Build history of the part. All positions in model axes, mm. Coordinates: 2 decimals unless noted, no trailing zeros. Order: outer loops, then holes, each group sorted by start corner. A loop starts at its lowest first (then second) coordinate and runs counter-clockwise, first axis right, second up. Notation, with made-up numbers: (-18.5, 31.25) - (-13.5, 31.25) arc R16 ccw to (-13.5, 39.25) - close; hole circle Ø11 at (14, 80). An arc over 180 degrees is marked (long way). Write each question's results on one line, items separated by ' | '.
from build123d import *

# Parameters (mm, degrees)
F0_W     = 152.4
F0_H     = 76.2
F1_DEPTH = 1.5875
F2_W     = 5.08
F2_H     = 50.8
F3_DEPTH = 25.4
F5_DEPTH = 25.4


# Not quite as in the source:
# - a length typed as a fraction of an inch, garbled in the dataset ("3 / 203.2 mm" for 3/8 in), is restored


with BuildPart() as f1:
    # F0 (on Front) → F1 (new body)
    with BuildSketch(Plane.XZ):
        Rectangle(F0_W, F0_H)
    extrude(amount=F1_DEPTH)

    # F2 (on face) → F3 (cut)
    with BuildSketch(Plane.XZ.offset(1.5875)):
        Rectangle(F2_W, F2_H)
    extrude(amount=-F3_DEPTH, mode=Mode.SUBTRACT)

    # F4 (on face) → F5 (cut)
    with BuildSketch(Plane.XZ.offset(1.5875)):
        with BuildLine():
            Line((2.54, -25.4), (-2.54, -25.4))
            ThreePointArc((-2.54, -25.4), (0, -27.94), (2.54, -25.4))
        make_face()
        with BuildLine():
            ThreePointArc((2.54, 25.4), (0, 27.94), (-2.54, 25.4))
            Line((-2.54, 25.4), (2.54, 25.4))
        make_face()
    extrude(amount=-F5_DEPTH, mode=Mode.SUBTRACT)


solid = f1.part
1. Band-saw the part on C-C on x = 0. Give the cut face in (y, z), then the cut area to 3 significant figures.
Solved:
outline: (-1.59, -38.1) - (0, -38.1) - (0, -27.94) - (-1.59, -27.94) - close; (-1.59, 27.94) - (0, 27.94) - (0, 38.1) - (-1.59, 38.1) - close | area: 32.3 mm2
2. Band-saw the part on A-A on y = -1. Give the cut face in (x, z).
Solved:
outline: (-76.2, -38.1) - (76.2, -38.1) - (76.2, 38.1) - (-76.2, 38.1) - close; hole (-2.54, -25.4) arc R2.54 ccw to (2.54, -25.4) - (2.54, 25.4) arc R2.54 ccw to (-2.54, 25.4) - close
3. Band-saw the part on B-B on z = -17. Give the cut face in (x, y).
Solved:
outline: (-76.2, -1.59) - (-2.54, -1.59) - (-2.54, 0) - (-76.2, 0) - close; (2.54, -1.59) - (76.2, -1.59) - (76.2, 0) - (2.54, 0) - close
4. Probe line 1 (X direction, y = -1.2, z = -3). List the from-to ranges inside material, lowest first.
Solved:
line 1: x = -76.2 to -2.54, 2.54 to 76.2
